Can you work these out from the model? Positions are in its coordinate system, mm. A direction names the side the tool comes from. Give positions to 0.01 mm unless a question says otherwise; leave off trailing zeros. Answer as CSV lines item,"result".
```python
from build123d import *

# Parameters (mm, degrees)
FILETE1_R = 2


with BuildPart() as part:
    # Esboço1 → Revolução1 (revolve)
    with BuildSketch(Plane.XY, mode=Mode.PRIVATE) as revolu_o1_sk:
        with BuildLine():
            Line((41.75, 0), (51.1, 0))
            Line((51.1, 0), (51.1, 4.3))
            ThreePointArc((51.1, 4.3), (47.074305061, 5.987281185), (42.970510206, 4.5))
            Line((42.970510206, 4.5), (40.1, 4.5))
            Line((40.1, 4.5), (40.1, 3.3))
            Line((40.1, 3.3), (41.75, 1))
            Line((41.75, 1), (41.75, 0))
        make_face()
    revolve(revolu_o1_sk.sketch.rotate(Axis((0, -31.918770764, 0), (0, 1, 0)), 90), axis=Axis((0, -31.918770764, 0), (0, 1, 0)))

    # Filete1
    filete1_edges = [part.edges().sort_by_distance(p)[0] for p in [
        (0, 1, 41.75),
    ]]
    fillet(filete1_edges, radius=FILETE1_R)


solid = part.part
```
1) If we mould it in two halves opening along X, with no side actions, what happens to faces 3 (the cylindrical face through (40.757, 0.176, 9.051)), 4 (the cylindrical face through (49.885, 2.18, 11.077)), 5 (the flat face through (0, 0, -42))? For each: +X half, -X half, draft (parallel to the pull), parting line (faces both ways), or undercut.
Answer block:
face 3,"undercut"
face 4,"parting line"
face 5,"draft"
2) I need wall thicknesses on line 1 along X through (y, z) = (0.35, 0); line 2 along X through (y, z) = (3.8, 0); line 3 along Y through (x, z) = (-34.5, 31). Which ranges of each line are inside material? Lowest first, please. Write a range as [from, to].
Answer block:
line 1,"[-51.1, -41.75], [41.75, 51.1]"
line 2,"[-51.1, -40.1], [40.1, 51.1]"
line 3,"[0, 5.96]"
3) I'm going to push flat-ended pins straight in: P1, Ø2, axis at x = 19.5, z = 33.5, coming from the +Y side; P2, Ø2, axis at x = -20.5, y = 2, coming from the -Z side; P3, Ø1.5, axis at y = 4.5, z = -29, coming from the -X side; P4, Ø1.5, axis at x = -23, z = -36, coming from the +Y side. Where does each tip first touch, or does it pass through?
Answer block:
P1,"through"
P2,"z = -47.23"
P3,"x = -42.56"
P4,"y = 4.89"
4) Which directions (+Z, -Z, +X, -X, +Y, -Y) give clear straight access to the entire face, cutting with the end or side of a thin tool? Please do faces 1 (the cylindrical face through (24.4, 3.89, 31.82)), 2 (the flat face through (-38.4, 4.5, -12.5)).
Answer block:
face 1,"+Y, -Y"
face 2,"+Y"
